Study the drawing (mm; zero at the part's minimum x, y, z) and answer. Coordinates: 2 decimals unless noted, no trailing zeros. Order: outer loops, then holes, each group sorted by start corner. A loop starts at its lowest first (then second) coordinate and runs counter-clockwise, first axis right, second up. Notation, with made-up numbers: (67.5, 3) -> (105.5, 3) arc R21 cw to (105.5, 10) -> close; hole circle Ø5 at (-18.75, 5). An arc over 180 degrees is marked (long way). Answer as CSV lines item,"result". Start each with the question number.
Item 1: Straight lines are drawn through the part: L1, parallel to X at y = 12, z = 6.5; L2, parallel to Y at x = 12, z = 3.5; L3, parallel to X at y = 6, z = 4.25. For each, find the intervals that lie inside material, in ascending order.
Item 2: Section D-D (z = 1.5) is taken. Write down the section's boundary in (x, y).
Item 3: Section B-B (x = 63.5) is taken. Write down the section's boundary in (y, z) (3 decimals).
Item 4: Section C-C (x = 13) is taken. Write down the section's boundary in (y, z) (3 decimals).
Item 5: Section A-A (y = 21.5) is taken. Write down the section's boundary in (x, z) (3 decimals), then the cut area to 3 significant figures.
Item 6: Each of these flat-tipped pins is pushed along its axis until it touches: pin 1 Ø1.5 at (y, z) = (5.5, 6.5) entering from +X (3 decimals); pin 2 Ø5 at (x, z) = (26.5, 2.5) entering from +Y (3 decimals); pin 3 Ø10 at (x, y) = (110.5, 18) entering from +Z. Where does it stop, or does it pass through?
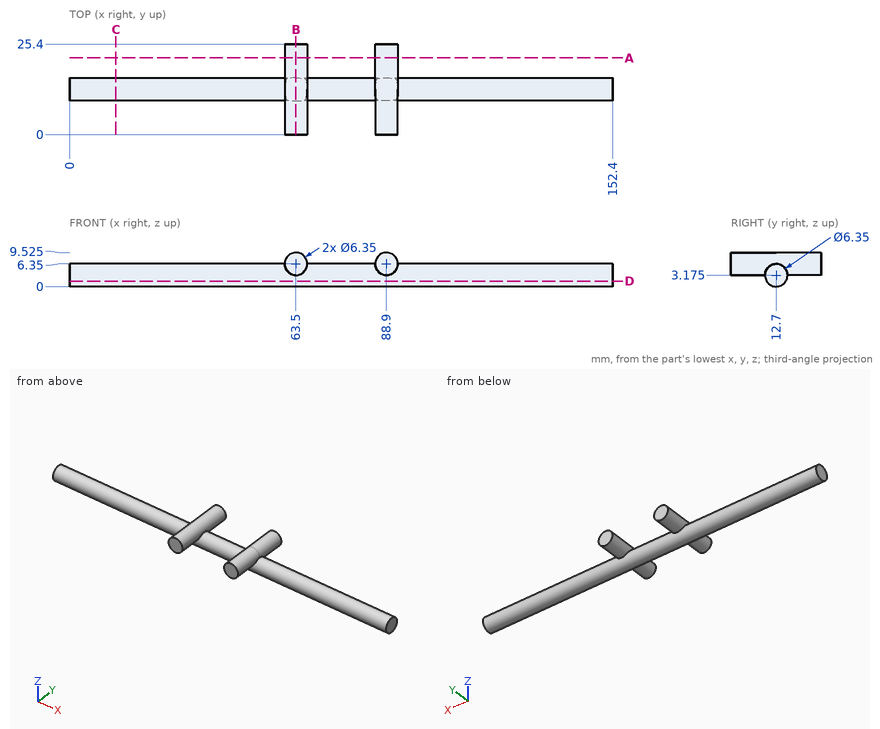
Checked values:
1,L1,"x = 60.33 to 66.67, 85.73 to 92.07"
1,L2,"y = 9.54 to 15.86"
1,L3,"x = 61.12 to 65.88, 86.52 to 91.28"
2,outline,"(0, 10) -> (152.4, 10) -> (152.4, 15.4) -> (0, 15.4) -> close"
3,outline,"(0, 3.175) -> (9.525, 3.175) arc R3.175 ccw to (15.875, 3.175) -> (25.4, 3.175) -> (25.4, 9.525) -> (0, 9.525) -> close"
4,outline,"circle Ø6.35 at (12.7, 3.175)"
5,outline,"circle Ø6.35 at (63.5, 6.35); circle Ø6.35 at (88.9, 6.35)"
5,area,"63.3 mm^2"
6,pin 1,"stops at x = 92.075"
6,pin 2,"stops at y = 15.875"
6,pin 3,"stops at z = 6.34"
